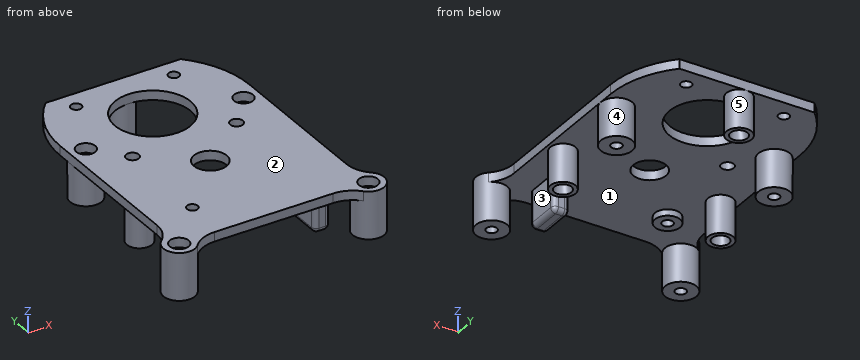
```python
from build123d import *

# Parameters (mm, degrees)
CYLINDER054_R               = 3
CYLINDER054_DEPTH           = 3
CYLINDER053_R               = 3
CYLINDER053_DEPTH           = 3
CYLINDER052_R               = 3
CYLINDER052_DEPTH           = 3
CYLINDER055_R               = 3
CYLINDER055_DEPTH           = 3
CYLINDER079_R               = 1.7
CYLINDER079_DEPTH           = 15
CYLINDER078_R               = 1.7
CYLINDER078_DEPTH           = 15
CYLINDER_R                  = 1.7
CYLINDER_DEPTH              = 15
CYLINDER080_R               = 1.7
CYLINDER080_DEPTH           = 15
CYLINDER107_R               = 1.7
CYLINDER107_DEPTH           = 5
CYLINDER086_R               = 5.2
CYLINDER086_DEPTH           = 3
BOX014_W                    = 44
BOX014_H                    = 10
BOX014_DEPTH                = 3
CYLINDER012_R               = 12
CYLINDER012_DEPTH           = 3
CYLINDER092_R               = 1.7
CYLINDER092_DEPTH           = 3
CYLINDER091_R               = 2
CYLINDER091_DEPTH           = 3
CYLINDER090_R               = 2
CYLINDER090_DEPTH           = 3
CYLINDER093_R               = 1.7
CYLINDER093_DEPTH           = 3
CYLINDER062_R               = 30
CYLINDER062_DEPTH           = 3
BOX018_W                    = 5
BOX018_H                    = 12
BOX018_DEPTH                = 14.5
FILLET011_R                 = 1.5
CYLINDER087_R               = 4
CYLINDER087_DEPTH           = 15
CYLINDER088_R               = 4
CYLINDER088_DEPTH           = 15
CYLINDER060_R               = 4
CYLINDER060_DEPTH           = 15
CYLINDER057_R               = 5
CYLINDER057_DEPTH           = 15
CYLINDER057_PLACEMENT_ANGLE = 215
CYLINDER056_R               = 5
CYLINDER056_DEPTH           = 15
CYLINDER056_PLACEMENT_ANGLE = -45
CYLINDER058_R               = 5
CYLINDER058_DEPTH           = 15
CYLINDER059_R               = 5
CYLINDER059_DEPTH           = 15
CYLINDER106_R               = 4
CYLINDER106_DEPTH           = 2
BOX008_W                    = 60
BOX008_H                    = 60
BOX008_DEPTH                = 3
FILLET014_R                 = 10


with BuildPart() as obj1:
    # Cylinder054 → Cylinder054 (new body)
    with BuildSketch(Plane(origin=(25, -5, 30), x_dir=(1, 0, 0), z_dir=(0, 0, 1))):
        Circle(CYLINDER054_R)
    extrude(amount=CYLINDER054_DEPTH)


with BuildPart() as obj2:
    # Cylinder053 → Cylinder053 (new body)
    with BuildSketch(Plane(origin=(-30, -60, 30), x_dir=(1, 0, 0), z_dir=(0, 0, 1))):
        Circle(CYLINDER053_R)
    extrude(amount=CYLINDER053_DEPTH)


with BuildPart() as obj3:
    # Cylinder052 → Cylinder052 (new body)
    with BuildSketch(Plane(origin=(30, -60, 30), x_dir=(1, 0, 0), z_dir=(0, 0, 1))):
        Circle(CYLINDER052_R)
    extrude(amount=CYLINDER052_DEPTH)


with BuildPart() as obj4:
    # Cylinder055 → Cylinder055 (new body)
    with BuildSketch(Plane(origin=(-25, -5, 30), x_dir=(1, 0, 0), z_dir=(0, 0, 1))):
        Circle(CYLINDER055_R)
    extrude(amount=CYLINDER055_DEPTH)

    # Fusion028: union obj1, obj2, obj3
    add(obj1.part)
    add(obj2.part)
    add(obj3.part)


with BuildPart() as obj5:
    # Cylinder079 → Cylinder079 (new body)
    with BuildSketch(Plane(origin=(25, -5, 18), x_dir=(1, 0, 0), z_dir=(0, 0, 1))):
        Circle(CYLINDER079_R)
    extrude(amount=CYLINDER079_DEPTH)


with BuildPart() as obj6:
    # Cylinder078 → Cylinder078 (new body)
    with BuildSketch(Plane(origin=(30, -60, 18), x_dir=(1, 0, 0), z_dir=(0, 0, 1))):
        Circle(CYLINDER078_R)
    extrude(amount=CYLINDER078_DEPTH)


with BuildPart() as obj7:
    # Cylinder → Cylinder (new body)
    with BuildSketch(Plane(origin=(-30, -60, 18), x_dir=(1, 0, 0), z_dir=(0, 0, 1))):
        Circle(CYLINDER_R)
    extrude(amount=CYLINDER_DEPTH)


with BuildPart() as obj8:
    # Cylinder080 → Cylinder080 (new body)
    with BuildSketch(Plane(origin=(-25, -5, 18), x_dir=(1, 0, 0), z_dir=(0, 0, 1))):
        Circle(CYLINDER080_R)
    extrude(amount=CYLINDER080_DEPTH)

    # Fusion027: union obj5, obj6, obj7
    add(obj5.part)
    add(obj6.part)
    add(obj7.part)


with BuildPart() as obj9:
    # Cone005 → Cone005 (revolve)
    with BuildSketch(Plane(origin=(-25, -32, 18), x_dir=(1, 0, 0), z_dir=(0, -1, 0))):
        Polygon((0, 0), (2.7, 0), (1.7, 5), (0, 5), align=None)
    revolve(axis=Axis((-25, -32, 18), (0, 0, 1)))


with BuildPart() as obj10:
    # Cone002 → Cone002 (revolve)
    with BuildSketch(Plane(origin=(0, 17, 18), x_dir=(1, 0, 0), z_dir=(0, -1, 0))):
        Polygon((0, 0), (2.7, 0), (1.7, 5), (0, 5), align=None)
    revolve(axis=Axis((0, 17, 18), (0, 0, 1)))


with BuildPart() as obj11:
    # Cone006 → Cone006 (revolve)
    with BuildSketch(Plane(origin=(25, -32, 18), x_dir=(1, 0, 0), z_dir=(0, -1, 0))):
        Polygon((0, 0), (2.7, 0), (1.7, 5), (0, 5), align=None)
    revolve(axis=Axis((25, -32, 18), (0, 0, 1)))

    # Fusion026: union obj9, obj10
    add(obj9.part)
    add(obj10.part)


with BuildPart() as obj12:
    # Cone011 → Cone011 (revolve)
    with BuildSketch(Plane(origin=(30, -60, 28.7), x_dir=(1, 0, 0), z_dir=(0, -1, 0))):
        Polygon((0, 0), (1.7, 0), (3, 1.3), (0, 1.3), align=None)
    revolve(axis=Axis((30, -60, 28.7), (0, 0, 1)))


with BuildPart() as obj13:
    # Cone010 → Cone010 (revolve)
    with BuildSketch(Plane(origin=(-30, -60, 28.7), x_dir=(1, 0, 0), z_dir=(0, -1, 0))):
        Polygon((0, 0), (1.7, 0), (3, 1.3), (0, 1.3), align=None)
    revolve(axis=Axis((-30, -60, 28.7), (0, 0, 1)))


with BuildPart() as obj14:
    # Cone009 → Cone009 (revolve)
    with BuildSketch(Plane(origin=(-25, -5, 28.7), x_dir=(1, 0, 0), z_dir=(0, -1, 0))):
        Polygon((0, 0), (1.7, 0), (3, 1.3), (0, 1.3), align=None)
    revolve(axis=Axis((-25, -5, 28.7), (0, 0, 1)))


with BuildPart() as obj15:
    # Cone008 → Cone008 (revolve)
    with BuildSketch(Plane(origin=(25, -5, 28.7), x_dir=(1, 0, 0), z_dir=(0, -1, 0))):
        Polygon((0, 0), (1.7, 0), (3, 1.3), (0, 1.3), align=None)
    revolve(axis=Axis((25, -5, 28.7), (0, 0, 1)))

    # Fusion031: union obj12, obj13, obj14
    add(obj12.part)
    add(obj13.part)
    add(obj14.part)


with BuildPart() as obj16:
    # Cylinder107 → Cylinder107 (new body)
    with BuildSketch(Plane(origin=(-17, -46, 28), x_dir=(1, 0, 0), z_dir=(0, 0, 1))):
        Circle(CYLINDER107_R)
    extrude(amount=CYLINDER107_DEPTH)


with BuildPart() as obj17:
    # Cylinder086 → Cylinder086 (new body)
    with BuildSketch(Plane(origin=(0, -28, 30), x_dir=(1, 0, 0), z_dir=(0, 0, 1))):
        Circle(CYLINDER086_R)
    extrude(amount=CYLINDER086_DEPTH)


with BuildPart() as obj18:
    # Box014 → Box014 (new body)
    with BuildSketch(Plane(origin=(-22, 21, 30), x_dir=(1, 0, 0), z_dir=(0, 0, 1))):
        with Locations((22, 5)):
            Rectangle(BOX014_W, BOX014_H)
    extrude(amount=BOX014_DEPTH)


with BuildPart() as obj19:
    # Cylinder012 → Cylinder012 (new body)
    with BuildSketch(Plane(origin=(0, 1, 30), x_dir=(1, 0, 0), z_dir=(0, 0, 1))):
        Circle(CYLINDER012_R)
    extrude(amount=CYLINDER012_DEPTH)


with BuildPart() as obj20:
    # Cylinder092 → Cylinder092 (new body)
    with BuildSketch(Plane(origin=(-15.5, 15, 30), x_dir=(1, 0, 0), z_dir=(0, 0, 1))):
        Circle(CYLINDER092_R)
    extrude(amount=CYLINDER092_DEPTH)


with BuildPart() as obj21:
    # Cylinder091 → Cylinder091 (new body)
    with BuildSketch(Plane(origin=(-16.5, -15, 30), x_dir=(1, 0, 0), z_dir=(0, 0, 1))):
        Circle(CYLINDER091_R)
    extrude(amount=CYLINDER091_DEPTH)


with BuildPart() as obj22:
    # Cylinder090 → Cylinder090 (new body)
    with BuildSketch(Plane(origin=(16.5, -15, 30), x_dir=(1, 0, 0), z_dir=(0, 0, 1))):
        Circle(CYLINDER090_R)
    extrude(amount=CYLINDER090_DEPTH)


with BuildPart() as obj23:
    # Cylinder093 → Cylinder093 (new body)
    with BuildSketch(Plane(origin=(15.5, 15, 30), x_dir=(1, 0, 0), z_dir=(0, 0, 1))):
        Circle(CYLINDER093_R)
    extrude(amount=CYLINDER093_DEPTH)

    # Fusion025: union obj20, obj21, obj22
    add(obj20.part)
    add(obj21.part)
    add(obj22.part)


with BuildPart() as cylinderbasetop:
    # Cylinder062 → Cylinder062 (new body)
    with BuildSketch(Plane.XY.offset(30)):
        Circle(CYLINDER062_R)
    extrude(amount=CYLINDER062_DEPTH)


with BuildPart() as slidingboxtop:
    # Box018 → Box018 (new body)
    with BuildSketch(Plane(origin=(16, -55, 18.5), x_dir=(1, 0, 0), z_dir=(0, 0, 1))):
        with Locations((2.5, 6)):
            Rectangle(BOX018_W, BOX018_H)
    extrude(amount=BOX018_DEPTH)

    # Fillet011
    fillet011_edges = [slidingboxtop.edges().sort_by_distance(p)[0] for p in [
        (16, -55, 25.75),
        (16, -43, 25.75),
        (16, -49, 18.5),
        (21, -55, 25.75),
        (21, -43, 25.75),
        (21, -49, 18.5),
        (18.5, -55, 18.5),
        (18.5, -43, 18.5),
    ]]
    fillet(fillet011_edges, radius=FILLET011_R)


with BuildPart() as cylinder114:
    # Cylinder087 → Cylinder087 (new body)
    with BuildSketch(Plane(origin=(25, -32, 18), x_dir=(1, 0, 0), z_dir=(0, 0, 1))):
        Circle(CYLINDER087_R)
    extrude(amount=CYLINDER087_DEPTH)


with BuildPart() as cylinder115:
    # Cylinder088 → Cylinder088 (new body)
    with BuildSketch(Plane(origin=(-25, -32, 18), x_dir=(1, 0, 0), z_dir=(0, 0, 1))):
        Circle(CYLINDER088_R)
    extrude(amount=CYLINDER088_DEPTH)


with BuildPart() as cylinderalignmentboltstop:
    # Cylinder060 → Cylinder060 (new body)
    with BuildSketch(Plane(origin=(0, 17, 18), x_dir=(1, 0, 0), z_dir=(0, 0, 1))):
        Circle(CYLINDER060_R)
    extrude(amount=CYLINDER060_DEPTH)

    # Fusion029: union Cylinder114, Cylinder115
    add(cylinder114.part)
    add(cylinder115.part)


with BuildPart() as cylinder049:
    # Cylinder057 → Cylinder057 (new body)
    with BuildSketch(Plane.XY):
        Circle(CYLINDER057_R)
    extrude(amount=CYLINDER057_DEPTH)


with BuildPart() as cylinder049_1:
    # Cylinder057 placement: moved
    add(cylinder049.part.moved(Location((-30, -60, 18))).rotate(Axis((-30, -60, 18), (0, 0, 1)), CYLINDER057_PLACEMENT_ANGLE))


with BuildPart() as cylinder048:
    # Cylinder056 → Cylinder056 (new body)
    with BuildSketch(Plane.XY):
        Circle(CYLINDER056_R)
    extrude(amount=CYLINDER056_DEPTH)


with BuildPart() as cylinder048_1:
    # Cylinder056 placement: moved
    add(cylinder048.part.moved(Location((30, -60, 18))).rotate(Axis((30, -60, 18), (0, 0, 1)), CYLINDER056_PLACEMENT_ANGLE))


with BuildPart() as cylinder050:
    # Cylinder058 → Cylinder058 (new body)
    with BuildSketch(Plane(origin=(25, -5, 18), x_dir=(1, 0, 0), z_dir=(0, 0, 1))):
        Circle(CYLINDER058_R)
    extrude(amount=CYLINDER058_DEPTH)


with BuildPart() as cylindernutstop:
    # Cylinder059 → Cylinder059 (new body)
    with BuildSketch(Plane(origin=(-25, -5, 18), x_dir=(1, 0, 0), z_dir=(0, 0, 1))):
        Circle(CYLINDER059_R)
    extrude(amount=CYLINDER059_DEPTH)

    # Fusion030: union Cylinder049, Cylinder048, Cylinder050
    add(cylinder049_1.part)
    add(cylinder048_1.part)
    add(cylinder050.part)


with BuildPart() as cylinderholderwashertop:
    # Cylinder106 → Cylinder106 (new body)
    with BuildSketch(Plane(origin=(-17, -46, 28), x_dir=(1, 0, 0), z_dir=(0, 0, 1))):
        Circle(CYLINDER106_R)
    extrude(amount=CYLINDER106_DEPTH)


with BuildPart() as extrudercasetop:
    # Box008 → Box008 (new body)
    with BuildSketch(Plane(origin=(-30, -60, 30), x_dir=(1, 0, 0), z_dir=(0, 0, 1))):
        with Locations((30, 30)):
            Rectangle(BOX008_W, BOX008_H)
    extrude(amount=BOX008_DEPTH)

    # Fusion037: union CylinderBaseTop, SlidingBoxTop, CylinderAlignmentBoltsTop, CylinderNutsTop, CylinderHolderWasherTop
    add(cylinderbasetop.part)
    add(slidingboxtop.part)
    add(cylinderalignmentboltstop.part)
    add(cylindernutstop.part)
    add(cylinderholderwashertop.part)

    # Cut073: cut obj23
    add(obj23.part, mode=Mode.SUBTRACT)

    # Cut074: cut obj19
    add(obj19.part, mode=Mode.SUBTRACT)

    # Cut075: cut obj18
    add(obj18.part, mode=Mode.SUBTRACT)

    # Cut076: cut obj17
    add(obj17.part, mode=Mode.SUBTRACT)

    # Cut077: cut obj16
    add(obj16.part, mode=Mode.SUBTRACT)

    # Cut078: cut obj15
    add(obj15.part, mode=Mode.SUBTRACT)

    # Cut079: cut obj11
    add(obj11.part, mode=Mode.SUBTRACT)

    # Cut080: cut obj8
    add(obj8.part, mode=Mode.SUBTRACT)

    # Cut081: cut obj4
    add(obj4.part, mode=Mode.SUBTRACT)

    # Fillet014
    fillet014_edges = [extrudercasetop.edges().sort_by_distance(p)[0] for p in [
        (30, -55, 31.5),
        (25, -60, 31.5),
        (-25, -60, 31.5),
        (-30, -55, 31.5),
    ]]
    fillet(fillet014_edges, radius=FILLET014_R)


solid = extrudercasetop.part
```
Input: part model. Units: mm. Frame: model coordinates. Face numbers are marked on the shaded views. A direction names the side the tool comes from. Round coordinates to 2 decimals unless told otherwise and drop trailing zeros. Order: outer loops, then holes, each group sorted by start corner. A loop starts at its lowest first (then second) coordinate and runs counter-clockwise, first axis right, second up. Notation, with made-up numbers: (11, 2) - (66, 2) arc R22 ccw to (66, 19) - close; hole circle Ø7 at (8, -21). An arc over 180 degrees is marked (long way). One line per question, with ' | ' between items. Start each with the question number.
1) Cut plane C-C, the plane x = -10. Return the cut outline in (y, z), then the cut area to 3 significant figures.
2) Contact query for flat-ended pins moving along their axis: P1, Ø3, axis at y = -49.5, z = 21.5, coming from the +X side; P2, Ø1.6, axis at x = 18, z = 24, coming from the +Y side; P3, Ø10, axis at x = -15, y = 9.5, coming from the -Z side. Output: stop coordinate, or through.
3) Cut plane A-A, the plane z = 25.75. Give the number of separate pieces and of enclosed holes in the cut face, then the cut area to 3 significant figures.
4) Set-up query: the marked faces 1 and 2. Return all of +Z, -Z, +X, -X, +Y, -Y with unobstructed straight access to the full face (end or side cutting, diameter ignored); none if empty.
5) Cut plane B-B, the plane y = -25. Return the cut outline in (x, z).
6) Pull-direction query (Y, two-part tool) for the marked faces 3, 4 and 5; classes: +Y half, -Y half, draft (parallel to the pull), parting line (faces both ways), or undercut.
7) Ray query, probe 1 along X at (y, z) = (-3.5, 28); probe 2 along X at (y, z) = (-6, 25.75); probe 3 along Y at (x, z) = (-25.5, 23.5). Return the intervals inside material, ascending.
Worked out:
1) outline: (-60, 30) - (-5.63, 30) - (-5.63, 33) - (-60, 33) - close; (7.63, 30) - (21, 30) - (21, 33) - (7.63, 33) - close | area: 203 mm^2
2) P1: stops at x = 21 | P2: stops at y = -43 | P3: stops at z = 30
3) separate pieces: 8 | enclosed holes: 4 | area: 487 mm^2
4) face 1: -Z | face 2: +Z, +X, -X, +Y, -Y
5) outline: (-30, 30) - (-4.25, 30) - (-4.25, 33) - (-30, 33) - close; (4.25, 30) - (30, 30) - (30, 33) - (4.25, 33) - close
6) face 3: draft | face 4: undercut | face 5: parting line
7) probe 1: x = -29.77 to -25.8, -24.2 to -20.23, 20.23 to 24.2, 25.8 to 29.77 | probe 2: x = -29.9 to -26.37, -23.63 to -20.1, 20.1 to 23.63, 26.37 to 29.9 | probe 3: y = -62.18 to -57.82, -35.97 to -28.03, -9.97 to -6.62, -3.38 to -0.03
